```python
from build123d import *

# Parameters (mm, degrees)
SKETCH1_R           = 21
SKETCH1_R_2         = 14.5
BOSS_EXTRUDE1_DEPTH = 2.5
CUT_EXTRUDE1_START  = -4
CUT_EXTRUDE1_DEPTH  = 4


with BuildPart() as part:
    # Sketch1 → Boss-Extrude1 (new body)
    with BuildSketch(Plane.XY):
        Circle(SKETCH1_R)
        Circle(SKETCH1_R_2, mode=Mode.SUBTRACT)
    extrude(amount=BOSS_EXTRUDE1_DEPTH)

    # Sketch2 → Cut-Extrude1 (cut)
    with BuildSketch(Plane.XY.offset(2.5).offset(CUT_EXTRUDE1_START)):
        with BuildLine():
            Line((0, 17), (0, 14.5))
            ThreePointArc((0, 14.5), (2.268299743, 14.321480939), (4.480746418, 13.790319486))
            Line((4.480746418, 13.790319486), (5.253288904, 16.167960777))
            ThreePointArc((5.253288904, 16.167960777), (2.659385906, 16.79070179), (0, 17))
        make_face()
        with BuildLine():
            Line((9.992349289, 13.753288904), (8.522886158, 11.730746418))
            ThreePointArc((8.522886158, 11.730746418), (10.253048327, 10.253048327), (11.730746418, 8.522886158))
            Line((11.730746418, 8.522886158), (13.753288904, 9.992349289))
            ThreePointArc((13.753288904, 9.992349289), (12.02081528, 12.02081528), (9.992349289, 13.753288904))
        make_face()
        with BuildLine():
            Line((16.167960777, 5.253288904), (13.790319486, 4.480746418))
            ThreePointArc((13.790319486, 4.480746418), (14.321480939, 2.268299743), (14.5, 0))
            Line((14.5, 0), (17, 0))
            ThreePointArc((17, 0), (16.79070179, 2.659385906), (16.167960777, 5.253288904))
        make_face()
        with BuildLine():
            Line((16.167960777, -5.253288904), (13.790319486, -4.480746418))
            ThreePointArc((13.790319486, -4.480746418), (12.919594601, -6.582862246), (11.730746418, -8.522886158))
            Line((11.730746418, -8.522886158), (13.753288904, -9.992349289))
            ThreePointArc((13.753288904, -9.992349289), (15.147110911, -7.717838496), (16.167960777, -5.253288904))
        make_face()
        with BuildLine():
            Line((9.992349289, -13.753288904), (8.522886158, -11.730746418))
            ThreePointArc((8.522886158, -11.730746418), (6.582862246, -12.919594601), (4.480746418, -13.790319486))
            Line((4.480746418, -13.790319486), (5.253288904, -16.167960777))
            ThreePointArc((5.253288904, -16.167960777), (7.717838496, -15.147110911), (9.992349289, -13.753288904))
        make_face()
        with BuildLine():
            Line((0, -17), (0, -14.5))
            ThreePointArc((0, -14.5), (-2.268299743, -14.321480939), (-4.480746418, -13.790319486))
            Line((-4.480746418, -13.790319486), (-5.253288904, -16.167960777))
            ThreePointArc((-5.253288904, -16.167960777), (-2.659385906, -16.79070179), (0, -17))
        make_face()
        with BuildLine():
            Line((-9.992349289, -13.753288904), (-8.522886158, -11.730746418))
            ThreePointArc((-8.522886158, -11.730746418), (-10.253048327, -10.253048327), (-11.730746418, -8.522886158))
            Line((-11.730746418, -8.522886158), (-13.753288904, -9.992349289))
            ThreePointArc((-13.753288904, -9.992349289), (-12.02081528, -12.02081528), (-9.992349289, -13.753288904))
        make_face()
        with BuildLine():
            Line((-16.167960777, -5.253288904), (-13.790319486, -4.480746418))
            ThreePointArc((-13.790319486, -4.480746418), (-14.321480939, -2.268299743), (-14.5, 0))
            Line((-14.5, 0), (-17, 0))
            ThreePointArc((-17, 0), (-16.79070179, -2.659385906), (-16.167960777, -5.253288904))
        make_face()
        with BuildLine():
            Line((-16.167960777, 5.253288904), (-13.790319486, 4.480746418))
            ThreePointArc((-13.790319486, 4.480746418), (-12.919594601, 6.582862246), (-11.730746418, 8.522886158))
            Line((-11.730746418, 8.522886158), (-13.753288904, 9.992349289))
            ThreePointArc((-13.753288904, 9.992349289), (-15.147110911, 7.717838496), (-16.167960777, 5.253288904))
        make_face()
        with BuildLine():
            Line((-9.992349289, 13.753288904), (-8.522886158, 11.730746418))
            ThreePointArc((-8.522886158, 11.730746418), (-6.582862246, 12.919594601), (-4.480746418, 13.790319486))
            Line((-4.480746418, 13.790319486), (-5.253288904, 16.167960777))
            ThreePointArc((-5.253288904, 16.167960777), (-7.717838496, 15.147110911), (-9.992349289, 13.753288904))
        make_face()
    extrude(amount=CUT_EXTRUDE1_DEPTH, mode=Mode.SUBTRACT)


solid = part.part
```
The listing builds one solid part. Answer for the finished solid, in the listing's coordinates (mm). Round coordinates to 2 decimals unless told otherwise and drop trailing zeros. Loops run counter-clockwise (first coordinate to the right, second up) from the corner with the lowest first, then second, coordinate; pieces in that order, holes last.
Q1. For a pull along X with two mould halves and no side action, classify faces 1 (the face through (-12.73, 9.25, 1.23)), 2 (the face through (14, 5, 0)) as released by +X, released by -X, zero draft, split by the parting line, or undercut.
Q2. Section C-C, the plane y = 1 is taken. Determine the outline of the cut face in (x, z), then the cut area to 3 significant figures.
Q3. Section B-B, the plane x = -1.5 is taken. Determine the outline of the cut face in (y, z).
Q4. Section D-D, the plane x = 17.5 is taken. Determine the outline of the cut face in (y, z).
Q5. Given pin 1 Ø1.2 at (x, z) = (15.5, 2) entering from +Y; pin 2 Ø1.5 at (y, z) = (16.5, 0.5) entering from -X; pin 3 Ø1.2 at (y, z) = (16, 1) entering from +X, each flat-ended and moving along its own axis, determine where each tip first touches the part or whether it passes through.
Q6. Find the intervals of material crossed by line 1 (X direction, y = 12.5, z = 0.9); line 2 (Y direction, x = -9.5, z = 1.9); line 3 (X direction, y = 4, z = 1.4), in increasing order.
Q7. Section A-A, the plane x = -15 is taken. Determine the outline of the cut face in (y, z), then the cut area to 3 significant figures.
Completed:
1. face 1: undercut
1. face 2: zero draft
2. outline: (-20.98, 0) - (-14.47, 0) - (-14.47, 2.5) - (-20.98, 2.5) - close; (16.97, 0) - (20.98, 0) - (20.98, 2.5) - (16.97, 2.5) - close
2. area: 26.3 mm2
3. outline: (-20.95, 0) - (-16.93, 0) - (-16.93, 2.5) - (-20.95, 2.5) - close; (14.42, 0) - (20.95, 0) - (20.95, 2.5) - (14.42, 2.5) - close
4. outline: (-11.61, 0) - (11.61, 0) - (11.61, 2.5) - (-11.61, 2.5) - close
5. pin 1: stops at y = 14.8
5. pin 2: stops at x = -13.89
5. pin 3: stops at x = 14.28
6. line 1: x = -16.87 to -9.08, 7.35 to 9.08, 11.52 to 16.87
6. line 2: y = -18.73 to -13.08, 10.95 to 13.08, 14.1 to 18.73
6. line 3: x = -20.62 to -13.94, 16.52 to 20.62
7. outline: (-14.7, 0) - (-4.87, 0) - (-4.87, 2.5) - (-14.7, 2.5) - close; (0, 0) - (4.87, 0) - (4.87, 2.5) - (0, 2.5) - close; (8, 0) - (14.7, 0) - (14.7, 2.5) - (8, 2.5) - close
7. area: 53.5 mm2
